Build history of the part. All positions in model axes, mm. A direction names the side the tool comes from. Give positions to 0.01 mm unless a question says otherwise; leave off trailing zeros. Loops run counter-clockwise (first coordinate to the right, second up) from the corner with the lowest first, then second, coordinate; pieces in that order, holes last.
1) Band-saw the part on D-D on y = 31. List the corners of the cut face in (x, z), then the cut area to 3 significant figures.
2) Wall check: line 1 (Y direction, x = 54, z = 2); line 2 (X direction, y = 49, z = 0.75); line 3 (Z direction, x = -16, y = 24.5). Give the ranges that are in metal, low to high.
3) Band-saw the part on B-B on x = -47.5. List the corners of the cut face in (y, z).
4) 3-axis set-ups, long thin cutter, end or side, ignore diameter. For faces 1 (the flat face through (-0.71, 56.4, 6.18)), 2 (the cylindrical face through (-56.248, -48.327, 1.479)), 3 (the flat face through (52, 52.128, 1)): which of +Z, -Z, +X, -X, +Y, -Y reach the whole face in a straight line?
5) Band-saw the part on C-C on x = 0. List the corners of the cut face in (y, z).
6) Flat gauge pins, fed straight in: P1, Ø5, axis at y = 54.5, z = 4.5, coming from the -X side; P2, Ø7, axis at x = -54, y = -48.228, coming from the +Z side; P3, Ø1.5, axis at x = -52.5, z = 1.5, coming from the +Y side. Where does each tip first touch, or does it go through?
7) Two-plate mould, pull along X, no slides. Class faces 4 (the flat face through (-57.9, -1, 1)), 5 (the flat face through (-53, 52.128, 1)), 6 (the cylindrical face through (51.752, -0.099, 1.479)): +X half, -X half, draft (parallel to the pull), parting line (faces both ways), or undercut.
8) Band-saw the part on A-A on y = 0. List the corners of the cut face in (x, z).
Autodesk Fusion 360 part; units mm, degrees
sketch "Sketch1" plane through (0, 0, 0) normal (0, 0, 1) x (1, 0, 0)
  line L0 (-57.9, 52.128) -> (57.9, 52.128)
  line L1 (57.9, 52.128) -> (57.9, -52.128)
  line L2 (57.9, -52.128) -> (-57.9, -52.128)
  line L3 (-57.9, -52.128) -> (-57.9, 52.128)
  circle A0 centre (-54, 48.228) radius 3.9
  circle A1 centre (-54, 0) radius 2.25
  circle A2 centre (-54, -48.228) radius 3.9
  circle A3 centre (0, -48.228) radius 2.25
  circle A4 centre (54, -48.228) radius 3.9
  circle A5 centre (54, 0) radius 2.25
  circle A6 centre (54, 48.228) radius 3.9
  circle A7 centre (-54, 48.228) radius 2.25
  circle A8 centre (-54, -48.228) radius 2.25
  circle A9 centre (54, -48.228) radius 2.25
  circle A10 centre (54, 48.228) radius 2.25
  point P0 (0, 52.128)
  point P1 (-57.9, 0)
  dimension "d1" = 115.8
  dimension "d2" = 104.256
  dimension "d3" = 7.8
  dimension "d4" = 7.8
  dimension "d5" = 7.8
  dimension "d6" = 7.8
  dimension "d7" = 4.5
  dimension "d8" = 4.5
  dimension "d9" = 4.5
  dimension "d10" = 4.5
  dimension "d11" = 4.5
  dimension "d12" = 4.5
  dimension "d13" = 4.5
  dimension "d14" = 48.128
  dimension "d15" = 96.256
  dimension "d16" = 53.9
  dimension "d17" = 107.8
extrude "Extrude1" add sketch "Sketch1" along normal blind 3 contours L0 L1 L2 L3 A0 A2 A4 A6 | A0 | A6 | A2 | A4
sketch "Sketch2" plane through (0, 0, 0) normal (1, 0, 0) x (0, 1, 0)
  line L0 (-2.25, 3) -> (2.25, 3)
  line L1 (-50.478, 3) -> (-45.978, 3)
  line L2 (-2.25, 3) -> (2.25, 3)
  line L3 (45.978, 3) -> (50.478, 3)
  line L4 (-50.478, 3) -> (-45.978, 3)
  line L5 (45.978, 3) -> (50.478, 3)
  line L6 (-50.478, 3) -> (-45.978, 3)
  line L7 (-48.228, 3) -> (-52.128, 3)
  line L8 (-48.228, 3) -> (48.228, 3)
  line L9 (52.128, 3) -> (48.228, 3)
  line L10 (52.128, 3) -> (48.228, 3)
  line L11 (48.228, 3) -> (-48.228, 3)
  line L12 (-48.228, 3) -> (-52.128, 3)
  line L13 (52.128, 0) -> (52.128, 3)
  line L14 (52.128, 3) -> (52.128, 0)
  line L15 (-2.25, 0) -> (2.25, 0)
  line L16 (-50.478, 0) -> (-45.978, 0)
  line L17 (-2.25, 0) -> (2.25, 0)
  line L18 (45.978, 0) -> (50.478, 0)
  line L19 (-50.478, 0) -> (-45.978, 0)
  line L20 (45.978, 0) -> (50.478, 0)
  line L21 (-50.478, 0) -> (-45.978, 0)
  line L22 (-48.228, 0) -> (-52.128, 0)
  line L23 (-48.228, 0) -> (-52.128, 0)
  line L24 (-48.228, 0) -> (48.228, 0)
  line L25 (52.128, 0) -> (48.228, 0)
  line L26 (52.128, 0) -> (48.228, 0)
  line L27 (48.228, 0) -> (-48.228, 0)
  line L28 (52.128, 3) -> (52.128, 6)
  line L29 (52.128, 6) -> (55.128, 6)
  line L30 (55.128, 6) -> (58.0826, 3.5208)
  line L31 (58.0826, 3.5208) -> (56.1543, 1.2226)
  line L32 (56.1543, 1.2226) -> (62.2826, -3.9197)
  line L33 (62.2826, -3.9197) -> (61.2567, -5.1423)
  line L34 (61.2567, -5.1423) -> (55.1284, 0)
  line L35 (56.1543, 1.2226) -> (55.1284, 0)
  line L36 (55.1284, 0) -> (52.128, 0)
  dimension "d20" = 3
  dimension "d21" = 3
  dimension "d22" = 140
  dimension "d24" = 3.857
  dimension "d26" = 3
  dimension "d27" = 8
  dimension "d28" = 1.596
extrude "Extrude2" add sketch "Sketch2" along normal mid plane 102 contours L13 L14 L28 L29 L30 L31 L35 L36
sketch "Sketch1 (2)" plane through (0, 25.732, 30.6662) normal (0, 0.6428, 0.766) x (-1, 0, 0)
  line L0 (51, -38.3738) -> (-51, -38.3738)
  line L1 (-51, -38.3738) -> (-51, -42.2308)
  line L2 (-51, -42.2308) -> (51, -42.2308)
  line L3 (51, -42.2308) -> (51, -38.3738)
  line L4 (51, -39.2308) -> (-51, -39.2308)
  line L5 (-51, -39.2308) -> (-51, -36.2308)
  line L6 (-51, -36.2308) -> (51, -36.2308)
  line L7 (51, -36.2308) -> (51, -39.2308)
  dimension "d67" = 3
  dimension "d68" = 3
extrude "Extrude4" add sketch "Sketch1 (2)" against normal blind 7 contours L0 L1 L3 L4 L5 L7 | L0 L5 L6 L7
sketch "Sketch2 (2)" plane through (0, 25.732, 30.6662) normal (0, 0.6428, 0.766) x (-1, 0, 0)
  line L0 (-51, -36.2308) -> (-51, -42.2308)
  line L1 (-51, -42.2308) -> (51, -42.2308)
  line L2 (51, -42.2308) -> (51, -36.2308)
  line L3 (51, -36.2308) -> (-51, -36.2308)
  line L4 (51, -39.2308) -> (-51, -39.2308)
  line L5 (-51, -39.2308) -> (-51, -36.2308)
  line L6 (-51, -36.2308) -> (51, -36.2308)
  line L7 (51, -36.2308) -> (51, -39.2308)
  dimension "d71" = 3
extrude "Extrude5" add sketch "Sketch2 (2)" along normal blind 6 contours L0 L2 L3 L4 L5 L6 L7
sketch "Sketch3" plane through (0, 30.0525, -25.2171) normal (0, 0.766, -0.6428) x (-1, 0, 0)
  line L0 (-51, 40.0319) -> (51, 40.0319)
  line L1 (51, 40.0319) -> (51, 46.0319)
  line L2 (51, 46.0319) -> (-51, 46.0319)
  line L3 (-51, 46.0319) -> (-51, 40.0319)
  circle A0 centre (0, 43.0319) radius 1.425
  dimension "d74" = 2.85
  dimension "d75" = 3
extrude "Extrude6" cut sketch "Sketch3" against normal blind 4 contours A0
equation "d4 = d3"
equation "d5 = d3"
equation "d6 = d3"
equation "d8 = d7"
equation "d9 = d7"
equation "d10 = d7"
equation "d11 = d7"
equation "d12 = d7"
equation "d13 = d7"
Findings below:
1. outline: (-57.9, 0) - (57.9, 0) - (57.9, 3) - (-57.9, 3) - close
1. area: 347 mm2
2. line 1: y = -52.13 to -50.48, -45.98 to -2.25, 2.25 to 45.98, 50.48 to 52.13
2. line 2: x = -57.82 to -56.11, -51.89 to 51.89, 56.11 to 57.82
2. line 3: z = 0 to 3
3. outline: (-52.13, 0) - (55.13, 0) - (56.15, 1.22) - (58.08, 3.52) - (55.78, 5.45) - (59.64, 10.05) - (57.34, 11.97) - (52.33, 6) - (52.13, 6) - (52.13, 5.76) - (49.81, 3) - (-52.13, 3) - close
4. face 1: +X, -X, +Y
4. face 2: +Z, -Z
4. face 3: +Z, -Z, +X, +Y
5. outline: (-52.13, 0) - (-50.48, 0) - (-50.48, 3) - (-52.13, 3) - close; (-45.98, 0) - (55.13, 0) - (56.15, 1.22) - (58.08, 3.52) - (55.78, 5.45) - (56.8, 6.66) - (54.5, 8.58) - (52.33, 6) - (52.13, 6) - (52.13, 5.76) - (49.81, 3) - (-45.98, 3) - close; (56.33, 10.77) - (58.63, 8.84) - (59.64, 10.05) - (57.34, 11.97) - close
6. P1: stops at x = -51
6. P2: stops at z = 3
6. P3: stops at y = 52.13
7. face 4: -X half
7. face 5: draft
7. face 6: undercut
8. outline: (-57.9, 0) - (-56.25, 0) - (-56.25, 3) - (-57.9, 3) - close; (-51.75, 0) - (51.75, 0) - (51.75, 3) - (-51.75, 3) - close; (56.25, 0) - (57.9, 0) - (57.9, 3) - (56.25, 3) - close
